```python
from build123d import *

# Parameters (mm, degrees)
PCB_DEPTH              = 1.6
MOUNT_HOLES_D          = 2.75
SKETCH5_W              = 17
SKETCH5_H              = 13.18
USB_HOST_DEPTH         = 15.5
SKETCH6_W              = 21.3
SKETCH6_H              = 16
ETHERNET_DEPTH         = 14.15
SKETCH7_W              = 3
SKETCH7_H              = 20.5
CAMERA_CONNECTOR_DEPTH = 5.5
SKETCH9_W              = 15
SKETCH9_H              = 11.5
HDMI_DEPTH             = 6.4
SKETCH10_W             = 7
SKETCH10_H             = 15
AV_DEPTH               = 5.8
SKETCH12_W             = 7.6
SKETCH12_H             = 5.6
USB_MICRO_DEPTH        = 2.5
SKETCH13_W             = 3
SKETCH13_H             = 20.5
DISPLAY_DEPTH          = 5.6
SKETCH14_W             = 50.8
SKETCH14_H             = 5
GPIO_DEPTH             = 8.54
SKETCH15_W             = 17
SKETCH15_H             = 11
USD_CARD_DEPTH         = 1


with BuildPart() as part:
    # Sketch2 → PCB (new body)
    with BuildSketch(Plane(origin=(0, 0, 0), x_dir=(1, 0, 0), z_dir=(0, 1, 0))):
        with BuildLine():
            Line((3, 0), (82, 0))
            ThreePointArc((82, 0), (84.121320344, 0.878679656), (85, 3))
            Line((85, 3), (85, 53))
            ThreePointArc((85, 53), (84.121320344, 55.121320344), (82, 56))
            Line((82, 56), (3, 56))
            ThreePointArc((3, 56), (0.878679656, 55.121320344), (0, 53))
            Line((0, 53), (0, 3))
            ThreePointArc((0, 3), (0.878679656, 0.878679656), (3, 0))
        make_face()
    extrude(amount=PCB_DEPTH)

    # Mount Holes (through all)
    with Locations(Plane(origin=(0, 1.6, 0), x_dir=(1, 0, 0), z_dir=(0, 1, 0))):
        with Locations((3.5, 3.5), (3.5, 52.5), (61.5, 52.5), (61.5, 3.5)):
            Hole(MOUNT_HOLES_D / 2)

    # Sketch5 → USB Host (add)
    with BuildSketch(Plane(origin=(0, 1.6, 0), x_dir=(1, 0, 0), z_dir=(0, 1, 0))):
        with Locations((78.5, 47)):
            Rectangle(SKETCH5_W, SKETCH5_H)
        with Locations((78.5, 29)):
            Rectangle(SKETCH5_W, SKETCH5_H)
    extrude(amount=USB_HOST_DEPTH)

    # Sketch6 → Ethernet (add)
    with BuildSketch(Plane(origin=(0, 1.6, 0), x_dir=(1, 0, 0), z_dir=(0, 1, 0))):
        with Locations((76.35, 10.25)):
            Rectangle(SKETCH6_W, SKETCH6_H)
    extrude(amount=ETHERNET_DEPTH)

    # Sketch7 → Camera Connector (add)
    with BuildSketch(Plane(origin=(0, 1.6, 0), x_dir=(1, 0, 0), z_dir=(0, 1, 0))):
        with Locations((45, 11.5)):
            Rectangle(SKETCH7_W, SKETCH7_H)
    extrude(amount=CAMERA_CONNECTOR_DEPTH)

    # Sketch9 → HDMI (add)
    with BuildSketch(Plane(origin=(0, 1.6, 0), x_dir=(1, 0, 0), z_dir=(0, 1, 0))):
        with Locations((32, 4.45)):
            Rectangle(SKETCH9_W, SKETCH9_H)
    extrude(amount=HDMI_DEPTH)

    # Sketch10 → AV (add)
    with BuildSketch(Plane(origin=(0, 1.6, 0), x_dir=(1, 0, 0), z_dir=(0, 1, 0))):
        with Locations((53.5, 5)):
            Rectangle(SKETCH10_W, SKETCH10_H)
    extrude(amount=AV_DEPTH)

    # Sketch12 → USB-Micro (add)
    with BuildSketch(Plane(origin=(0, 1.6, 0), x_dir=(1, 0, 0), z_dir=(0, 1, 0))):
        with Locations((10.6, 1.7)):
            Rectangle(SKETCH12_W, SKETCH12_H)
    extrude(amount=USB_MICRO_DEPTH)

    # Sketch13 → Display (add)
    with BuildSketch(Plane(origin=(0, 1.6, 0), x_dir=(1, 0, 0), z_dir=(0, 1, 0))):
        with Locations((3.8, 28)):
            Rectangle(SKETCH13_W, SKETCH13_H)
    extrude(amount=DISPLAY_DEPTH)

    # Sketch14 → GPIO (add)
    with BuildSketch(Plane(origin=(0, 1.6, 0), x_dir=(1, 0, 0), z_dir=(0, 1, 0))):
        with Locations((32.5, 52.7)):
            Rectangle(SKETCH14_W, SKETCH14_H)
    extrude(amount=GPIO_DEPTH)

    # Sketch15 → uSD Card (add)
    with BuildSketch(Plane.XZ):
        with Locations((5.5, -27.5)):
            Rectangle(SKETCH15_W, SKETCH15_H)
    extrude(amount=USD_CARD_DEPTH)


solid = part.part
```
Verification items for the finished model (mm, model axes). A direction names the side the tool comes from. Give positions to 0.01 mm unless a question says otherwise; leave off trailing zeros. Write each loop counter-clockwise with the first axis right and the second up, starting at its lowest first coordinate (ties: lowest second). Pieces come first, ordered by that corner, then holes. Notation, with made-up numbers: (72.25, 82) - (92.25, 82) arc R15 ccw to (92.25, 86) - close; hole circle Ø8 at (52.5, 89.25). An arc over 180 degrees is marked (long way). Put each result on its own line as item: value.
Q1. Section check C-C on y = 5.5. Count the separate pieces of the cut face and the enclosed holes in it, and give its area (3 significant figures).
Result:
separate pieces: 8
enclosed holes: 0
area: 1,440 mm2
Q2. Set-up check for faces 1 (the face through (4, 4, -17.75)), 2 (the face through (78, 9, -22.41)), 3 (the face through (53, 4, -12.5)): record each of +Z, -Z, +X, -X, +Y, -Y from which the full face is reachable in a straight line by a thin tool's end or side.
Result:
face 1: +Z, -X, +Y
face 2: +X, +Y
face 3: +Y
Q3. Depth check by flat-ended pin: P1, Ø8, axis at x = 30, z = -6.5, coming from the -Y side; P2, Ø2, axis at x = 3.5, z = -52.5, coming from the +Y side; P3, Ø5, axis at x = 52, y = 10, coming from the +Z side; P4, Ø4.5, axis at y = 5.5, z = -15, coming from the -X side. Enter the tip coordinate at first touch or a pass-through.
Result:
P1: y = 0
P2: through
P3: z = -50.2
P4: x = 43.5
Q4. Scan lines: probe 1 along X at (y, z) = (1.1, -52.5) (3 decimals); probe 2 along Z at (x, y) = (3.5, 0.65) (3 decimals); probe 3 along X at (y, z) = (3.75, -28.5). Record each from-to range of solid material in increasing order. Write a range as from..to.
Result:
probe 1: 0..2.125, 4.875..60.125, 62.875..85
probe 2: -56..-53.875, -51.125..-4.875, -2.125..0
probe 3: 2.3..5.3, 70..87
Q5. Mould release check, pull along Z, two halves, no side actions. Record for faces 4 (the face through (45, 7.1, -12)), 5 (the face through (4, 4, -38.25)), 6 (the face through (2.87, 0.79, -2.28)): released by +Z, released by -Z, zero draft, split by the parting line, or undercut.
Result:
face 4: zero draft
face 5: released by -Z
face 6: undercut
Q6. Section check A-A on y = 14. Record the cut outline in (x, z), and give its area (3 significant figures).
Result:
outline: (65.7, -18.25) - (87, -18.25) - (87, -2.25) - (65.7, -2.25) - close; (70, -53.59) - (87, -53.59) - (87, -40.41) - (70, -40.41) - close; (70, -35.59) - (87, -35.59) - (87, -22.41) - (70, -22.41) - close
area: 789 mm2
Q7. Section check B-B on x = 61.5. Record the cut outline in (y, z) (3 decimals).
Result:
outline: (0, -56) - (1.6, -56) - (1.6, -53.875) - (0, -53.875) - close; (0, -51.125) - (1.6, -51.125) - (1.6, -4.875) - (0, -4.875) - close; (0, -2.125) - (1.6, -2.125) - (1.6, 0) - (0, 0) - close
Q8. Section check D-D on z = -32. Record the cut outline in (x, y), and give its area (3 significant figures).
Result:
outline: (-3, -1) - (14, -1) - (14, 0) - (85, 0) - (85, 1.6) - (87, 1.6) - (87, 17.1) - (70, 17.1) - (70, 1.6) - (5.3, 1.6) - (5.3, 7.2) - (2.3, 7.2) - (2.3, 1.6) - (0, 1.6) - (0, 0) - (-3, 0) - close
area: 433 mm2
